Model file for the job. Use its own axes, mm. Face numbers are marked on the shaded views. A direction names the side the tool comes from. Round coordinates to 2 decimals unless told otherwise and drop trailing zeros. Write each loop counter-clockwise with the first axis right and the second up, starting at its lowest first coordinate (ties: lowest second). Pieces come first, ordered by that corner, then holes.
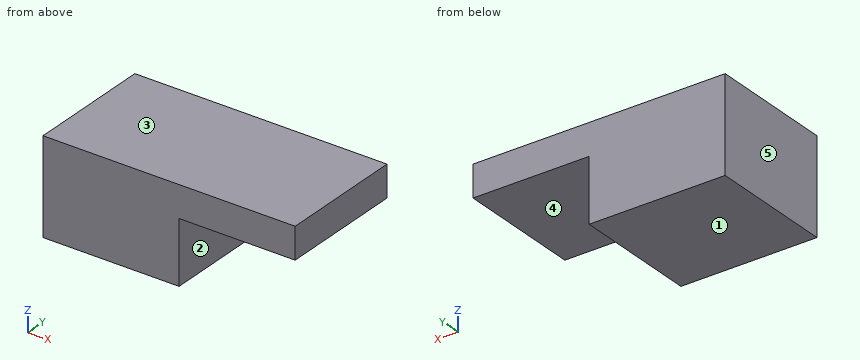
```python
from build123d import *

# Parameters (mm, degrees)
F0_W     = 21.585796
F0_H     = 20
F1_DEPTH = 10
F2_W     = 18.414204
F2_H     = 20
F2_W_2   = 21.585796
F3_DEPTH = 5


with BuildPart() as f1:
    # F0 (on Top) → F1 (new body)
    with BuildSketch(Plane.XY):
        Rectangle(F0_W, F0_H)
    extrude(amount=F1_DEPTH)

    # F2 (on face) → F3 (join)
    with BuildSketch(Plane.XY.offset(10)):
        with Locations((20, 0)):
            Rectangle(F2_W, F2_H)
        Rectangle(F2_W_2, F2_H)
    extrude(amount=F3_DEPTH)


solid = f1.part
```
1) Cut at B-B on x = 15.5. List the corners of the cut face in (y, z).
2) Pull direction Z, two halves, no side cores. Call the marked faces 1, 2 and 3: released by +Z, released by -Z, zero draft, split by the parting line, or undercut.
3) Flat gauge pin, fed straight in: pin 1 Ø6 at (y, z) = (-5.5, 6.5) entering from +X. Where does the tip first touch, or does it go through?
4) Which spindle directions (+Z, -Z, +X, -X, +Y, -Y) get a long thin tool onto all of the face, cutting with end or side? Do the marked faces 4 and 5. Say none if no direction does.
5) Cut at A-A on y = -6. List the corners of the cut face in (x, z), and give its area (3 significant figures).
6) Cut at C-C on z = 4. List the corners of the cut face in (x, y), and give its area (3 significant figures).
7) Wall check: probe 1 along X at (y, z) = (4, 2.25); probe 2 along Z at (x, y) = (18, -2). Give the ranges that are in metal, low to high.
Result sheet:
1. outline: (-10, 10) - (10, 10) - (10, 15) - (-10, 15) - close
2. face 1: released by -Z
2. face 2: zero draft
2. face 3: released by +Z
3. pin 1: stops at x = 10.79
4. face 4: -Z, +X, +Y, -Y
4. face 5: +Z, -Z, -X, +Y, -Y
5. outline: (-10.79, 0) - (10.79, 0) - (10.79, 10) - (29.21, 10) - (29.21, 15) - (-10.79, 15) - close
5. area: 416 mm2
6. outline: (-10.79, -10) - (10.79, -10) - (10.79, 10) - (-10.79, 10) - close
6. area: 432 mm2
7. probe 1: x = -10.79 to 10.79
7. probe 2: z = 10 to 15
